Geometry: final body of the model. Coordinates: model frame, mm. A direction names the side the tool comes from. Round coordinates to 2 decimals unless told otherwise and drop trailing zeros. Loops run counter-clockwise (first coordinate to the right, second up) from the corner with the lowest first, then second, coordinate; pieces in that order, holes last. Notation, with made-up numbers: (73.25, 49) - (128.25, 49) arc R12 ccw to (128.25, 55) - close; hole circle Ø1 at (9.5, 21). An arc over 180 degrees is marked (long way). Use CSV: the item, a comma, the result in double quotes.
Autodesk Inventor part; units mm, degrees
ref_plane "YZ Plane" through (0, 0, 0) normal (1, 0, 0) x (0, 1, 0)
ref_plane "XZ Plane" through (0, 0, 0) normal (0, 1, 0) x (-1, 0, 0)
ref_plane "XY Plane" through (0, 0, 0) normal (0, 0, 1) x (1, 0, 0)
sketch "Sketch1" plane through (0, 0, 0) normal (0, 1, 0) x (-1, 0, 0)
  line L0 (-158.7435, 10.9468) -> (-196.8435, 10.9468)
  line L1 (-196.8435, 10.9468) -> (-196.8435, 87.1468)
  line L2 (-196.8435, 87.1468) -> (-158.7435, 87.1468)
  line L3 (-158.7435, 87.1468) -> (-158.7435, 10.9468)
  line L4 (-161.9185, 83.9718) -> (-193.6685, 83.9718)
  line L5 (-193.6685, 83.9718) -> (-193.6685, 14.1218)
  line L6 (-193.6685, 14.1218) -> (-161.9185, 14.1218)
  line L7 (-161.9185, 14.1218) -> (-161.9185, 83.9718)
  point P0 (0, 0)
  dimension "d0" = 76.2
  dimension "d1" = 38.1
  dimension "d2" = 3.175
extrude "Extrusion1" add sketch "Sketch1" along normal blind 114.3
sketch "Sketch2" plane through (158.7435, 0, 87.1468) normal (0, 0, 1) x (1, 0, 0)
  line L0 (0, 0) -> (0, 114.3)
  line L1 (38.1, 0) -> (0, 0)
  point P0 (-158.7435, 0)
  point P1 (13.46, 8.89)
  point P2 (13.46, 21.59)
  point P3 (13.46, 34.29)
  point P4 (13.46, 46.99)
  point P5 (13.46, 59.69)
  point P6 (13.46, 72.39)
  point P7 (13.46, 85.09)
  point P8 (13.46, 97.79)
  dimension "d5" = 13.46
  dimension "d6" = 8.89
  dimension "d9" = 12.7
hole "Hole1" at (172.2035, 8.89, 87.1468) at (172.2035, 21.59, 87.1468) at (172.2035, 34.29, 87.1468) at (172.2035, 46.99, 87.1468) at (172.2035, 59.69, 87.1468) at (172.2035, 72.39, 87.1468) at (172.2035, 85.09, 87.1468) at (172.2035, 97.79, 87.1468) direction (0, 0, -1) diameter 5.08 end through all
properties part number "2018 Scissor Standoff Iner"
Item 1: Section D-D on y = 59.69. Return the cut outline in (x, z), plus the area to 3 significant figures.
Final values:
outline,"(158.74, 10.95) - (169.66, 10.95) - (169.66, 14.12) - (161.92, 14.12) - (161.92, 83.97) - (169.66, 83.97) - (169.66, 87.15) - (158.74, 87.15) - close; (174.74, 10.95) - (196.84, 10.95) - (196.84, 87.15) - (174.74, 87.15) - (174.74, 83.97) - (193.67, 83.97) - (193.67, 14.12) - (174.74, 14.12) - close"
area,"653 mm²"
Item 2: Section B-B on y = 86. Return the cut outline in (x, z).
Final values:
outline,"(158.74, 10.95) - (169.83, 10.95) - (169.83, 14.12) - (161.92, 14.12) - (161.92, 83.97) - (169.83, 83.97) - (169.83, 87.15) - (158.74, 87.15) - close; (174.57, 10.95) - (196.84, 10.95) - (196.84, 87.15) - (174.57, 87.15) - (174.57, 83.97) - (193.67, 83.97) - (193.67, 14.12) - (174.57, 14.12) - close"
Item 3: Section C-C on x = 179. Return the cut outline in (y, z), plus the area to 3 significant figures.
Final values:
outline,"(0, 10.95) - (114.3, 10.95) - (114.3, 14.12) - (0, 14.12) - close; (0, 83.97) - (114.3, 83.97) - (114.3, 87.15) - (0, 87.15) - close"
area,"726 mm²"
Item 4: Material intervals for line 1 (X direction, y = 35.5, z = 77); line 2 (Z direction, x = 184, y = 12); line 3 (X direction, y = 34.29, z = 85.5), sorted ascending.
Final values:
line 1,"x = 158.74 to 161.92, 193.67 to 196.84"
line 2,"z = 10.95 to 14.12, 83.97 to 87.15"
line 3,"x = 158.74 to 169.66, 174.74 to 196.84"
Item 5: Reachability of faces 1 (the flat face through (161.918, 56, 49)), 2 (the cylindrical face through (173.749, 87.106, 85.537)) from +Z, -Z, +X, -X, +Y, -Y: full face, straight path, thin tool, end or side. Return the list, or none.
Final values:
face 1,"+Y, -Y"
face 2,"+Z, -Z"
Item 6: Section A-A on z = 79. Return the cut outline in (x, y).
Final values:
outline,"(158.74, 0) - (161.92, 0) - (161.92, 114.3) - (158.74, 114.3) - close; (193.67, 0) - (196.84, 0) - (196.84, 114.3) - (193.67, 114.3) - close"
Item 7: Mould query, pull axis Z, two halves, no side actions, for faces 3 (the flat face through (193.668, 56, 50)), 4 (the cylindrical face through (174.46, 20.42, 85.54)), 5 (the flat face through (178, 56, 87.147)). Classes: released by +Z, released by -Z, zero draft, split by the parting line, or undercut.
Final values:
face 3,"undercut"
face 4,"zero draft"
face 5,"released by +Z"
